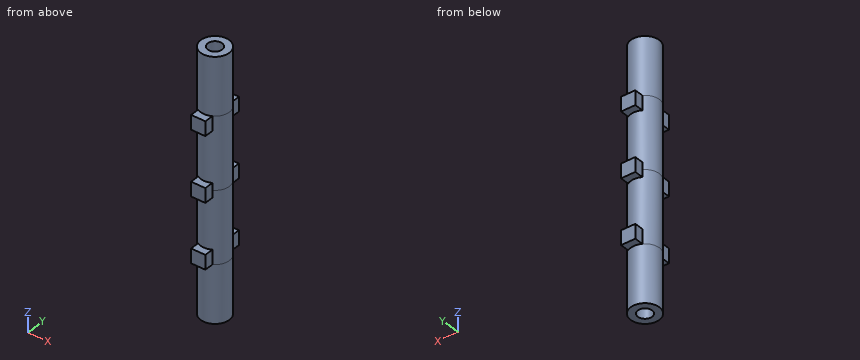
from build123d import *

# Parameters (mm, degrees)
SKETCH1_R             = 5
BOSS_EXTRUDE1_DEPTH   = 25
SKETCH2_W             = 5
SKETCH2_H             = 15
BOSS_EXTRUDE2_DEPTH   = 5
SKETCH3_W             = 5
SKETCH3_H             = 15
BOSS_EXTRUDE3_DEPTH   = 2.5
SKETCH5_W             = 5
SKETCH5_H             = 15
BOSS_EXTRUDE5_DEPTH   = 2.5
BOSS_EXTRUDE6_START   = 25
SKETCH6_R             = 5
BOSS_EXTRUDE6_DEPTH   = 25
SKETCH7_W             = 5
SKETCH7_H             = 15
BOSS_EXTRUDE7_DEPTH   = 5
F_5_0MM_DOWEL_HOLE1_D = 5
BOSS_EXTRUDE8_START   = 20
SKETCH14_R            = 5
BOSS_EXTRUDE8_DEPTH   = 20
SKETCH15_R            = 5
BOSS_EXTRUDE9_DEPTH   = 20
F_5_0MM_DOWEL_HOLE2_D = 5


with BuildPart() as part:
    # Sketch1 → Boss-Extrude1 (new body)
    with BuildSketch(Plane.XY):
        with Locations(Location((0, 0, 0), (0, 0, 180))):
            Circle(SKETCH1_R)
    extrude(amount=BOSS_EXTRUDE1_DEPTH)

    # Sketch2 → Boss-Extrude2 (add)
    with BuildSketch(Plane.XY.offset(25)):
        Rectangle(SKETCH2_W, SKETCH2_H)
    extrude(amount=-BOSS_EXTRUDE2_DEPTH)

    # Sketch3 → Boss-Extrude3 (add)
    with BuildSketch(Plane(origin=(0, 0, 0), x_dir=(-1, 0, 0), z_dir=(0, 0, -1))):
        Rectangle(SKETCH3_W, SKETCH3_H)
    extrude(amount=-BOSS_EXTRUDE3_DEPTH)

    # Sketch5 → Boss-Extrude5 (add)
    with BuildSketch(Plane(origin=(0, 0, 0), x_dir=(-1, 0, 0), z_dir=(0, 0, -1))):
        Rectangle(SKETCH5_W, SKETCH5_H)
    extrude(amount=BOSS_EXTRUDE5_DEPTH)

    # Sketch6 → Boss-Extrude6 (add)
    with BuildSketch(Plane(origin=(0, 0, 0), x_dir=(-1, 0, 0), z_dir=(0, 0, -1)).offset(BOSS_EXTRUDE6_START)):
        Circle(SKETCH6_R)
    extrude(amount=-BOSS_EXTRUDE6_DEPTH)

    # Sketch7 → Boss-Extrude7 (add)
    with BuildSketch(Plane(origin=(0, 0, -25), x_dir=(-1, 0, 0), z_dir=(0, 0, -1))):
        Rectangle(SKETCH7_W, SKETCH7_H)
    extrude(amount=-BOSS_EXTRUDE7_DEPTH)

    # Ø5.0mm Dowel Hole1 (through all)
    with Locations(Plane.XY.offset(25)):
        with Locations((0, 0)):
            Hole(F_5_0MM_DOWEL_HOLE1_D / 2)

    # Sketch14 → Boss-Extrude8 (add)
    with BuildSketch(Plane(origin=(0, 0, -25), x_dir=(-1, 0, 0), z_dir=(0, 0, -1)).offset(BOSS_EXTRUDE8_START)):
        Circle(SKETCH14_R)
    extrude(amount=-BOSS_EXTRUDE8_DEPTH)

    # Sketch15 → Boss-Extrude9 (add)
    with BuildSketch(Plane.XY.offset(25)):
        with Locations(Location((0, 0, 0), (0, 0, 180))):
            Circle(SKETCH15_R)
    extrude(amount=BOSS_EXTRUDE9_DEPTH)

    # Ø5.0mm Dowel Hole2 (through all)
    with Locations(Plane(origin=(0, 0, -45), x_dir=(-1, 0, 0), z_dir=(0, 0, -1))):
        with Locations((0, 0)):
            Hole(F_5_0MM_DOWEL_HOLE2_D / 2)


solid = part.part
Read the model definition and answer for the solid it produces. Units are mm, in the model's axes. Coordinates: 2 decimals unless noted, no trailing zeros. Order: outer loops, then holes, each group sorted by start corner. A loop starts at its lowest first (then second) coordinate and runs counter-clockwise, first axis right, second up. Notation, with made-up numbers: (41.5, 57) -> (95.5, 57) arc R31 cw to (95.5, 89) -> close; hole circle Ø1 at (-21.75, -20.75). An arc over 180 degrees is marked (long way). Answer as a JSON object with one key per item and string values.
1) A cutting plane is placed at B-B, the plane z = -23.5. Determine the outline of the cut face in (x, y), plus the area to 3 significant figures.
Model answer:
{"outline": "(-2.5, -7.5) -> (2.5, -7.5) -> (2.5, -4.33) arc R5 ccw to (2.5, 4.33) -> (2.5, 7.5) -> (-2.5, 7.5) -> (-2.5, 4.33) arc R5 ccw to (-2.5, -4.33) -> close; hole circle Ø5 at (0, 0)", "area": "86.1 mm²"}
2) Each of these flat-tipped pins is pushed along its axis until it touches: pin 1 (3 mm diameter, centred on x = 0, y = 0, fed in from +Z); pin 2 (3.5 mm diameter, centred on y = 6, z = 23.5, fed in from -X); pin 3 (2.5 mm diameter, centred on x = 1, y = -6, fed in from +Z); pin 4 (8 mm diameter, centred on y = 5.5, z = -28.5, fed in from -X). Where does it stop, or does it pass through?
Model answer:
{"pin 1": "passes through", "pin 2": "stops at x = -2.63", "pin 3": "stops at z = 45", "pin 4": "stops at x = -4.77"}
3) A cutting plane is placed at D-D, the plane x = 4. Determine the outline of the cut face in (y, z).
Model answer:
{"outline": "(-3, -45) -> (3, -45) -> (3, 45) -> (-3, 45) -> close"}
4) A cutting plane is placed at A-A, the plane y = -6.5. Determine the outline of the cut face in (x, z), plus the area to 3 significant figures.
Model answer:
{"outline": "(-2.5, -25) -> (2.5, -25) -> (2.5, -20) -> (-2.5, -20) -> close; (-2.5, -2.5) -> (2.5, -2.5) -> (2.5, 2.5) -> (-2.5, 2.5) -> close; (-2.5, 20) -> (2.5, 20) -> (2.5, 25) -> (-2.5, 25) -> close", "area": "75.0 mm²"}
5) Consider line 1 along Y through (x, z) = (0, -29); line 2 along Z through (x, y) = (1.75, 6.75). Determine where each line is inside the solid, lowest interval first. Write a range as from..to.
Model answer:
{"line 1": "y = -5..-2.5, 2.5..5", "line 2": "z = -25..-20, -2.5..2.5, 20..25"}
